The listing builds one solid part. Answer for the finished solid, in the listing's coordinates (mm). A direction names the side the tool comes from. Round coordinates to 2 decimals unless told otherwise and drop trailing zeros. Loops run counter-clockwise (first coordinate to the right, second up) from the corner with the lowest first, then second, coordinate; pieces in that order, holes last. Notation, with made-up numbers: (71.25, -4) -> (102.25, -4) arc R22 cw to (102.25, 27) -> close; hole circle Ø8 at (64.5, 87). An arc over 180 degrees is marked (long way). Use a Markdown table: item, result. Add a question column.
Q1. Section C-C on z = 3 is taken. Give the vertices of the cut face in (x, y), then the cut area to 3 significant figures.
Q2. Given pin 1 Ø7.5 at (x, y) = (-30, -22.5) entering from +Z; pin 2 Ø4.5 at (x, y) = (-28, 35.5) entering from +Z, each flat-ended and moving along its own axis, determine where each tip first touches the part or whether it passes through.
Q3. Section B-B on y = -37.5 is taken. Give the vertices of the cut face in (x, z).
Q4. For a pull along Y with two mould halves and no side action, classify faces 1 (the flat face through (-1, -60, 13)), 2 (the flat face through (-1, 1, 25.4)), 3 (the cylindrical face through (15.44, 25.87, 12.52)), 4 (the cylindrical face through (-14.56, 25.87, 12.52)) as released by +Y, released by -Y, zero draft, split by the parting line, or undercut.
Q5. Section D-D on x = -32.5 is taken. Give the vertices of the cut face in (y, z).
Q6. Which of the six approach directions +Z, -Z, +X, -X, +Y, -Y give full straight-line access (tool end or side, diameter ignored) to faces 5 (the flat face through (33, -26, 15.87)), 6 (the cylindrical face through (-29.1, -26.53, 7.82))?
Q7. Section A-A on y = -22.5 is taken. Give the vertices of the cut face in (x, z).
Q8. Consider line 1 (Y direction, x = 30, z = 21.25); line 2 (Y direction, x = 15, z = 15.5); line 3 (X direction, y = 41, z = 11.5). Determine where each line is inside the solid, lowest interval first.
from build123d import *

# Parameters (mm, degrees)
F0_W           = 105
F0_H           = 120
F1_DEPTH       = 25.4
F3_D           = 8.26
F3_CBORE_D     = 14.5
F3_CBORE_DEPTH = 9.53
F5_D           = 6.8


with BuildPart() as f1:
    # F0 (on Top) → F1 (new body)
    with BuildSketch(Plane.XY):
        Rectangle(F0_W, F0_H)
    extrude(amount=F1_DEPTH)

    # F3 (through all)
    with Locations(Plane.XY.offset(25.4)):
        with Locations((-30, 37.5), (30, 37.5), (30, -22.5), (-30, -22.5)):
            CounterBoreHole(F3_D / 2, F3_CBORE_D / 2, F3_CBORE_DEPTH)

    # F5 (through all)
    with Locations(Plane.XY.offset(25.4)):
        with Locations((15, -37.5), (15, 22.5), (-15, 22.5)):
            Hole(F5_D / 2)


solid = f1.part
Checked values:
| question | item | result |
|---|---|---|
| 1 | outline | (-52.5, -60) -> (52.5, -60) -> (52.5, 60) -> (-52.5, 60) -> close; hole circle Ø8.26 at (-30, -22.5); hole circle Ø8.26 at (-30, 37.5); hole circle Ø6.8 at (-15, 22.5); hole circle Ø6.8 at (15, -37.5); hole circle Ø6.8 at (15, 22.5); hole circle Ø8.26 at (30, -22.5); hole circle Ø8.26 at (30, 37.5) |
| 1 | area | 12,300 mm2 |
| 2 | pin 1 | passes through |
| 2 | pin 2 | stops at z = 15.87 |
| 3 | outline | (-52.5, 0) -> (11.6, 0) -> (11.6, 25.4) -> (-52.5, 25.4) -> close; (18.4, 0) -> (52.5, 0) -> (52.5, 25.4) -> (18.4, 25.4) -> close |
| 4 | face 1 | released by -Y |
| 4 | face 2 | zero draft |
| 4 | face 3 | undercut |
| 4 | face 4 | undercut |
| 5 | outline | (-60, 0) -> (-25.79, 0) -> (-25.79, 15.87) -> (-29.31, 15.87) -> (-29.31, 25.4) -> (-60, 25.4) -> close; (-19.21, 0) -> (34.21, 0) -> (34.21, 15.87) -> (30.69, 15.87) -> (30.69, 25.4) -> (-15.69, 25.4) -> (-15.69, 15.87) -> (-19.21, 15.87) -> close; (40.79, 0) -> (60, 0) -> (60, 25.4) -> (44.31, 25.4) -> (44.31, 15.87) -> (40.79, 15.87) -> close |
| 6 | face 5 | +Z |
| 6 | face 6 | +Z, -Z |
| 7 | outline | (-52.5, 0) -> (-34.13, 0) -> (-34.13, 15.87) -> (-37.25, 15.87) -> (-37.25, 25.4) -> (-52.5, 25.4) -> close; (-25.87, 0) -> (25.87, 0) -> (25.87, 15.87) -> (22.75, 15.87) -> (22.75, 25.4) -> (-22.75, 25.4) -> (-22.75, 15.87) -> (-25.87, 15.87) -> close; (34.13, 0) -> (52.5, 0) -> (52.5, 25.4) -> (37.25, 25.4) -> (37.25, 15.87) -> (34.13, 15.87) -> close |
| 8 | line 1 | y = -60 to -29.75, -15.25 to 30.25, 44.75 to 60 |
| 8 | line 2 | y = -60 to -40.9, -34.1 to 19.1, 25.9 to 60 |
| 8 | line 3 | x = -52.5 to -32.19, -27.81 to 27.81, 32.19 to 52.5 |
